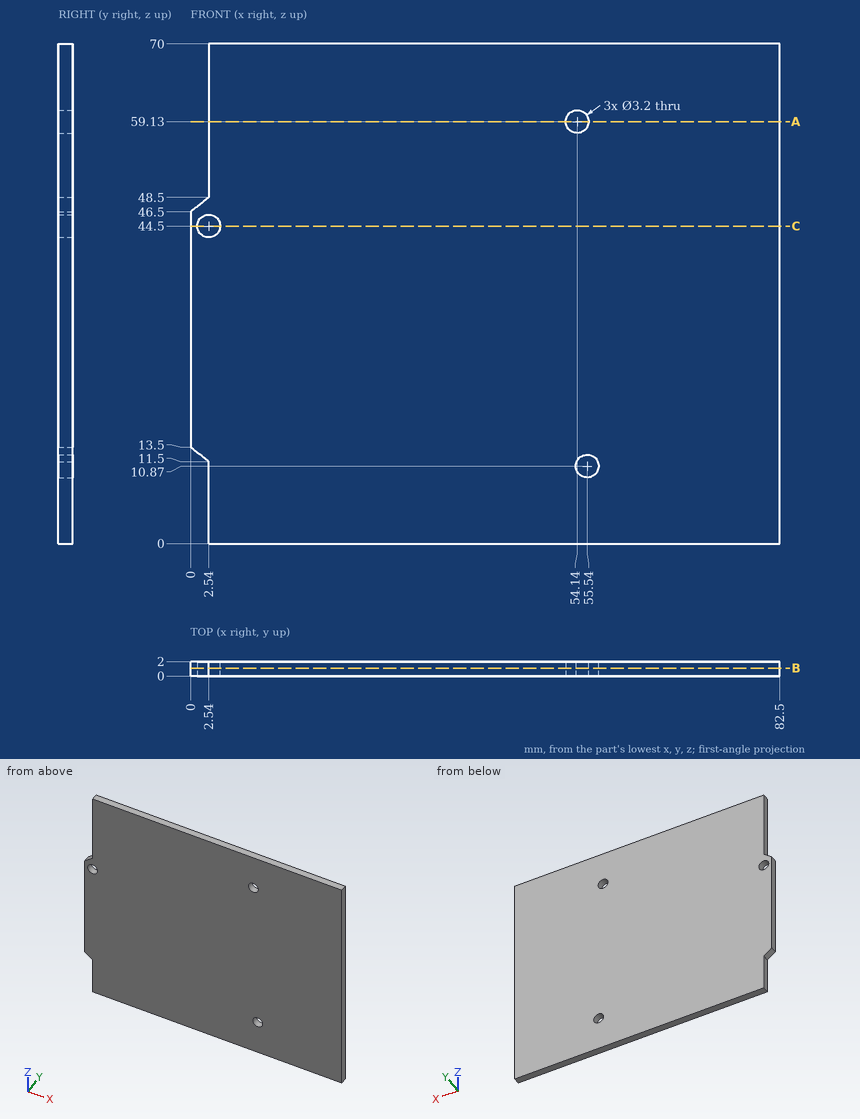
Print and shaded views of the part. All mm, measured from the part's lowest x, y and z. Give positions to 0.01 mm unless a question says otherwise; leave off trailing zeros. Loops run counter-clockwise (first coordinate to the right, second up) from the corner with the lowest first, then second, coordinate; pieces in that order, holes last.
1) Saw through at C-C (z = 44.5). Write the cut outline in (x, y), plus the area to 3 significant figures.
2) Flat gauge pins, fed straight in: pin 1 Ø1 at (y, z) = (0.5, 12) entering from -X; pin 2 Ø2.5 at (x, z) = (55.54, 10.87) entering from +Y; pin 3 Ø0.6 at (y, z) = (0.5, 5.5) entering from -X. Where does each tip first touch, or does it go through?
3) Saw through at B-B (y = 1.1). Write the cut outline in (x, z), plus the area to 3 significant figures.
4) Wall check: line 1 (Z direction, x = 55, y = 0.45); line 2 (X direction, y = 1.9, z = 50.5); line 3 (X direction, y = 0.95, z = 59.5). Give the ranges that are in metal, low to high.
5) Saw through at A-A (z = 59.13). Write the cut outline in (x, y), plus the area to 3 significant figures.
Answer block:
1. outline: (0, 0) - (0.94, 0) - (0.94, 2) - (0, 2) - close; (4.14, 0) - (82.5, 0) - (82.5, 2) - (4.14, 2) - close
1. area: 159 mm2
2. pin 1: stops at x = 1.27
2. pin 2: passes through
2. pin 3: stops at x = 2.54
3. outline: (0, 13.5) - (2.54, 11.5) - (2.54, 0) - (82.5, 0) - (82.5, 70) - (2.54, 70) - (2.54, 48.5) - (0, 46.5) - close; hole circle Ø3.2 at (2.54, 44.5); hole circle Ø3.2 at (54.14, 59.13); hole circle Ø3.2 at (55.54, 10.87)
3. area: 5,660 mm2
4. line 1: z = 0 to 9.36, 12.38 to 57.78, 60.48 to 70
4. line 2: x = 2.54 to 82.5
4. line 3: x = 2.54 to 52.58, 55.7 to 82.5
5. outline: (2.54, 0) - (52.54, 0) - (52.54, 2) - (2.54, 2) - close; (55.74, 0) - (82.5, 0) - (82.5, 2) - (55.74, 2) - close
5. area: 154 mm2
